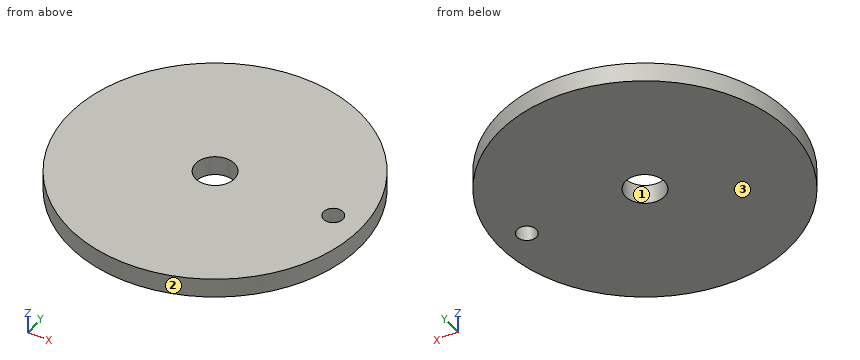
```python
from build123d import *

# Parameters (mm, degrees)
SKETCH1_R           = 1
BOSS_EXTRUDE1_DEPTH = 15
SKETCH2_R           = 7.5
BOSS_EXTRUDE2_DEPTH = 1
SKETCH3_R           = 0.5
CUT_EXTRUDE1_DEPTH  = 10
SKETCH5_R           = 1
CUT_EXTRUDE2_DEPTH  = 20


with BuildPart() as part:
    # Sketch1 → Boss-Extrude1 (new body)
    with BuildSketch(Plane.XY):
        Circle(SKETCH1_R)
    extrude(amount=BOSS_EXTRUDE1_DEPTH)

    # Sketch2 → Boss-Extrude2 (add)
    with BuildSketch(Plane.XY.offset(15)):
        Circle(SKETCH2_R)
    extrude(amount=BOSS_EXTRUDE2_DEPTH)

    # Sketch3 → Cut-Extrude1 (cut)
    with BuildSketch(Plane.XY.offset(16)):
        with Locations((6, 0)):
            Circle(SKETCH3_R)
    extrude(amount=-CUT_EXTRUDE1_DEPTH, mode=Mode.SUBTRACT)

    # Sketch5 → Cut-Extrude2 (cut)
    with BuildSketch(Plane.XY.offset(16)):
        Circle(SKETCH5_R)
    extrude(amount=-CUT_EXTRUDE2_DEPTH, mode=Mode.SUBTRACT)


solid = part.part
```
Could you check a few things on this model? Use its own coordinates, in mm. Face numbers are marked on the shaded views. Round coordinates to 2 decimals unless told otherwise and drop trailing zeros. Loops run counter-clockwise (first coordinate to the right, second up) from the corner with the lowest first, then second, coordinate; pieces in that order, holes last. Notation, with made-up numbers: M -5.5,6 L 19.5,6 A23 ccw 19.5,25 Z; hole C 4,-17.75 d1. An arc over 180 degrees is marked long. Write item = value, one per line.
1. Thinking about a two-plate mould opening in X: for the marked faces 1, 2 and 3, which applies, +X half, -X half, draft (parallel to the pull), parting line (faces both ways), or undercut?
Results below:
face_1 = undercut
face_2 = parting line
face_3 = draft
2. I want a section at C-C, the plane x = 6. Write out the boundary of the cut face in (y, z), and give its area (3 significant figures).
Results below:
outline = M -4.5,15 L -0.5,15 L -0.5,16 L -4.5,16 Z; M 0.5,15 L 4.5,15 L 4.5,16 L 0.5,16 Z
area = 8.00 mm²
3. I want a section at A-A, the plane x = 0. Write out the boundary of the cut face in (y, z), and give its area (3 significant figures).
Results below:
outline = M -7.5,15 L -1,15 L -1,16 L -7.5,16 Z; M 1,15 L 7.5,15 L 7.5,16 L 1,16 Z
area = 13.0 mm²
4. I need wall thicknesses on probe 1 along Y at (x, z) = (0, 15.5); probe 2 along Y at (x, z) = (6, 15.35); probe 3 along X at (y, z) = (2, 15.6). Which ranges of each line are inside material? Lowest first, please.
Results below:
probe_1 = -7.5 to -1, 1 to 7.5
probe_2 = -4.5 to -0.5, 0.5 to 4.5
probe_3 = -7.23 to 7.23
5. I want a section at D-D, the plane z = 15.55. Write out the boundary of the cut face in (x, y).
Results below:
outline = C 0,0 d15; hole C 0,0 d2; hole C 6,0 d1
6. I want a section at B-B, the plane y = 0. Write out the boundary of the cut face in (x, z).
Results below:
outline = M -7.5,15 L -1,15 L -1,16 L -7.5,16 Z; M 1,15 L 5.5,15 L 5.5,16 L 1,16 Z; M 6.5,15 L 7.5,15 L 7.5,16 L 6.5,16 Z
